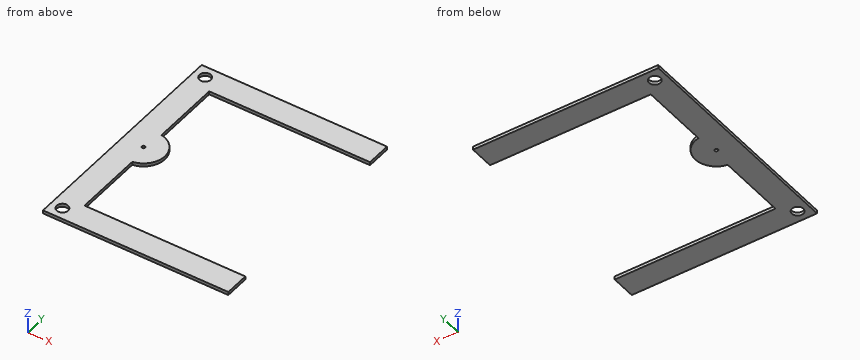
Autodesk Inventor part; units mm, degrees
ref_plane "YZ Plane" through (0, 0, 0) normal (1, 0, 0) x (0, 1, 0)
ref_plane "XZ Plane" through (0, 0, 0) normal (0, 1, 0) x (-1, 0, 0)
ref_plane "XY Plane" through (0, 0, 0) normal (0, 0, 1) x (1, 0, 0)
sketch "Boceto1" plane through (0, 0, 0) normal (0, 0, 1) x (1, 0, 0)
  circle A0 centre (32.0216, 148.5297) radius 3.5
  line L0 (40.0216, 140.5297) -> (40.0216, 98.3749)
  line L1 (40.0216, 72.6844) -> (40.0216, 30.5297)
  line L2 (25.0216, 15.5297) -> (25.0216, 155.5297)
  line L3 (40.0216, 30.5297) -> (138.3848, 30.5297)
  line L4 (6.0787, 0.7542) -> (6.0787, 166.9226)
  line L5 (163.6392, 166.9226) -> (163.6392, 0.7542)
  line L6 (138.3848, 15.5297) -> (25.0216, 15.5297)
  line L7 (163.6392, 0.7542) -> (6.0787, 0.7542)
  arc A1 (40.0216, 72.6844) -> (40.0216, 98.3749) centre (38.0216, 85.5297) ccw
  line L8 (138.3848, 30.5297) -> (138.3848, 15.5297)
  line L9 (138.3848, 155.5297) -> (138.3848, 140.5297)
  line L10 (138.3848, 140.5297) -> (40.0216, 140.5297)
  line L11 (6.0787, 166.9226) -> (163.6392, 166.9226)
  line L12 (25.0216, 155.5297) -> (138.3848, 155.5297)
  circle A2 centre (32.0216, 22.5297) radius 3.5
  circle A3 centre (38.0216, 85.5297) radius 1
  point P0 (0, 0)
  point P1 (0, 0)
  point P2 (40.0216, 98.3749)
  dimension "d0" = 2
extrude "Extrusión1" add sketch "Boceto1" along normal blind 2 contours L0 A1 L1 L3 L8 L6 L2 L12 L9 L10
properties part number "P8"
Here's how the part is built. I have some questions about the finished solid (model axes, mm). Round coordinates to 2 decimals unless told otherwise and drop trailing zeros. Order: outer loops, then holes, each group sorted by start corner. A loop starts at its lowest first (then second) coordinate and runs counter-clockwise, first axis right, second up. Notation, with made-up numbers: (78, -4.5) -> (89, -4.5) arc R7 ccw to (89, 0.5) -> close; hole circle Ø10 at (58, 71.5). An arc over 180 degrees is marked (long way). Use a Markdown table: item, result. Add a question column.
(1) Suppose I cut it at A-A, the plane x = 98. Please give me the cut outline in (y, z), and give its area (3 significant figures).
(2) Suppose I cut it at D-D, the plane y = 92. Please give me the cut outline in (x, z), and give its area (3 significant figures).
(3) Suppose I cut it at B-B, the plane z = 0.45. Please give me the cut outline in (x, y), and give its area (3 significant figures).
(4) Suppose I cut it at C-C, the plane y = 116.5. Please give me the cut outline in (x, z), and give its area (3 significant figures).
(5) I need wall thicknesses on line 1 along Y through (x, z) = (68.5, 0.5); line 2 along Y through (x, z) = (47, 1.2); line 3 along Y through (x, z) = (41, 1.1). Which ranges of each line are inside material? Lowest first, please.
(6) For pin 1 Ø5.5 at (x, y) = (32.02, 148.53) entering from +Z; pin 2 Ø1 at (y, z) = (44.5, 1.5) entering from +X, each with a flat end and sliding along its axis, tell me the tip position at first contact or that it passes through.
Verdict:
| question | item | result |
|---|---|---|
| 1 | outline | (15.53, 0) -> (30.53, 0) -> (30.53, 2) -> (15.53, 2) -> close; (140.53, 0) -> (155.53, 0) -> (155.53, 2) -> (140.53, 2) -> close |
| 1 | area | 60.0 mm2 |
| 2 | outline | (25.02, 0) -> (49.3, 0) -> (49.3, 2) -> (25.02, 2) -> close |
| 2 | area | 48.6 mm2 |
| 3 | outline | (25.02, 15.53) -> (138.38, 15.53) -> (138.38, 30.53) -> (40.02, 30.53) -> (40.02, 72.68) arc R13 ccw to (40.02, 98.37) -> (40.02, 140.53) -> (138.38, 140.53) -> (138.38, 155.53) -> (25.02, 155.53) -> close; hole circle Ø7 at (32.02, 22.53); hole circle Ø7 at (32.02, 148.53); hole circle Ø2 at (38.02, 85.53) |
| 3 | area | 5,180 mm2 |
| 4 | outline | (25.02, 0) -> (40.02, 0) -> (40.02, 2) -> (25.02, 2) -> close |
| 4 | area | 30.0 mm2 |
| 5 | line 1 | 15.53 to 30.53, 140.53 to 155.53 |
| 5 | line 2 | 15.53 to 30.53, 76.13 to 94.93, 140.53 to 155.53 |
| 5 | line 3 | 15.53 to 30.53, 72.88 to 98.18, 140.53 to 155.53 |
| 6 | pin 1 | through |
| 6 | pin 2 | x = 40.02 |
